Autodesk Inventor part; units mm, degrees
ref_plane "YZ Plane" through (0, 0, 0) normal (1, 0, 0) x (0, 1, 0)
ref_plane "XZ Plane" through (0, 0, 0) normal (0, 1, 0) x (-1, 0, 0)
ref_plane "XY Plane" through (0, 0, 0) normal (0, 0, 1) x (1, 0, 0)
sketch "Sketch1" plane through (0, 0, 0) normal (0, 0, 1) x (1, 0, 0)
  line L0 (0, 0) -> (25.4, 0)
  line L1 (25.4, 0) -> (25.4, 50.8)
  line L2 (25.4, 50.8) -> (0, 50.8)
  line L3 (0, 50.8) -> (0, 0)
  line L4 (2.54, 2.54) -> (22.86, 2.54)
  line L5 (22.86, 2.54) -> (22.86, 48.26)
  line L6 (22.86, 48.26) -> (2.54, 48.26)
  line L7 (2.54, 48.26) -> (2.54, 2.54)
  dimension "d0" = 25.4
  dimension "d1" = 50.8
  dimension "d2" = 20.32
  dimension "d3" = 45.72
  dimension "d4" = 2.54
  dimension "d5" = 2.54
extrude "Extrusion1" add sketch "Sketch1" along normal blind 254
sketch "Sketch2" plane through (0, 50.8, 0) normal (0, 1, 0) x (1, 0, 0)
  line L0 (25.4, 0) -> (0, 0)
  line L1 (0, 0) -> (0, -254)
  line L2 (25.4, -254) -> (0, -254)
  line L3 (25.4, 0) -> (25.4, -254)
  point P0 (12.7, -12.7)
  dimension "d8" = 12.7
  dimension "d9" = 12.7
hole "Hole1" at (12.7, 50.8, 12.7) direction (0, -1, 0) diameter 3.9688 end through all
pattern_linear "Rectangular Pattern1" count 10 spacing 25.4 along (0, 0, 1) of "Hole1"
sketch "Sketch3" plane through (0, 50.8, 0) normal (0, 1, 0) x (1, 0, 0)
  circle A0 centre (12.7, -241.3) radius 1.9844
  circle A1 centre (12.7, -215.9) radius 1.9844
  circle A2 centre (12.7, -190.5) radius 1.9844
  circle A3 centre (12.7, -165.1) radius 1.9844
  circle A4 centre (12.7, -139.7) radius 1.9844
  circle A5 centre (12.7, -114.3) radius 1.9844
  circle A6 centre (12.7, -88.9) radius 1.9844
  circle A7 centre (12.7, -63.5) radius 1.9844
  circle A8 centre (12.7, -38.1) radius 1.9844
  circle A9 centre (12.7, -12.7) radius 1.9844
  line L0 (25.4, 0) -> (0, 0)
  line L1 (0, 0) -> (0, -254)
  line L2 (25.4, -254) -> (0, -254)
  line L3 (25.4, 0) -> (25.4, -254)
  circle A10 centre (12.7, -12.7) radius 3.175
  circle A11 centre (12.7, -241.3) radius 3.175
  dimension "d20" = 6.35
  dimension "d21" = 6.35
extrude "Extrusion2" cut sketch "Sketch3" against normal blind 279.4 contours A0 | A9 | A10 | A11
sketch "Sketch4" plane through (25.4, 0, 0) normal (1, 0, 0) x (0, 0, -1)
  line L0 (0, 0) -> (0, 50.8)
  line L1 (0, 50.8) -> (-254, 50.8)
  line L2 (-254, 0) -> (-254, 50.8)
  line L3 (0, 0) -> (-254, 0)
  point P0 (-88.9, 38.1)
  dimension "d24" = 12.7
  dimension "d25" = 165.1
hole "Hole2" at (25.4, 38.1, 88.9) direction (-1, 0, 0) diameter 7.9375 end through all
properties part number "frame_side_bumper"
Could you check a few things on this model? Use its own coordinates, in mm. A direction names the side the tool comes from. Round coordinates to 2 decimals unless told otherwise and drop trailing zeros. Order: outer loops, then holes, each group sorted by start corner. A loop starts at its lowest first (then second) coordinate and runs counter-clockwise, first axis right, second up. Notation, with made-up numbers: M 41.5,36.25 L 82.5,36.25 A12 ccw 82.5,56.25 Z; hole C -8.5,24.5 d10. An arc over 180 degrees is marked long. One line per question, with ' | ' between items. Start each with the question number.
(1) Suppose I cut it at B-B on x = 4.75. List the corners of the cut face in (y, z) for me, then the cut area to 3 significant figures.
(2) Suppose I cut it at A-A on y = 13. List the corners of the cut face in (x, z) for me, then the cut area to 3 significant figures.
(3) Please list where these lines run through material, in increasing order: line 1 along Y through (x, z) = (7, 136); line 2 along X through (y, z) = (7.5, 53); line 3 along X through (y, z) = (1, 165).
(4) For faces 4 (the face through (14, 1, 189)), 5 (the face through (13, 2.54, 125)), which set-ups out of +Z, -Z, +X, -X, +Y, -Y let a thin tool reach every point of the face, with its end or its side?
(5) Suppose I cut it at C-C on z = 12.7. List the corners of the cut face in (x, y) for me (3 decimals), then the cut area to 3 significant figures.
(6) Suppose I cut it at D-D on y = 38.1. List the corners of the cut face in (x, z) for me, then the cut area to 3 significant figures.
(7) For P1, Ø2.5, axis at x = 12.7, z = 114.3, coming from the -Y side, with a flat end and sliding along its axis, tell me the tip position at first contact or that it passes through.
(8) Thinking about a two-plate mould opening in Z: for faces 1 (the face through (13.46, 1.252, 166.933)), 2 (the face through (13, 0, 125)), 3 (the face through (2, 27, 254)), which applies, +Z half, -Z half, draft (parallel to the pull), parting line (faces both ways), or undercut?
Geometry results:
1) outline: M 0,0 L 2.54,0 L 2.54,254 L 0,254 Z; M 48.26,0 L 50.8,0 L 50.8,254 L 48.26,254 Z | area: 1,290 mm²
2) outline: M 0,0 L 2.54,0 L 2.54,254 L 0,254 Z; M 22.86,0 L 25.4,0 L 25.4,254 L 22.86,254 Z | area: 1,290 mm²
3) line 1: 0 to 2.54, 48.26 to 50.8 | line 2: 0 to 2.54, 22.86 to 25.4 | line 3: 0 to 10.72, 14.68 to 25.4
4) face 4: +Y, -Y | face 5: +Z, -Z
5) outline: M 0,0 L 9.525,0 L 9.525,2.54 L 2.54,2.54 L 2.54,48.26 L 9.525,48.26 L 9.525,50.8 L 0,50.8 Z; M 15.875,0 L 25.4,0 L 25.4,50.8 L 15.875,50.8 L 15.875,48.26 L 22.86,48.26 L 22.86,2.54 L 15.875,2.54 Z | area: 329 mm²
6) outline: M 0,0 L 2.54,0 L 2.54,84.93 L 0,84.93 Z; M 0,92.87 L 2.54,92.87 L 2.54,254 L 0,254 Z; M 22.86,0 L 25.4,0 L 25.4,84.93 L 22.86,84.93 Z; M 22.86,92.87 L 25.4,92.87 L 25.4,254 L 22.86,254 Z | area: 1,250 mm²
7) P1: through
8) face 1: undercut | face 2: draft | face 3: +Z half
